Verification items for the finished model (mm, model axes). A direction names the side the tool comes from. Round coordinates to 2 decimals unless told otherwise and drop trailing zeros. Write each loop counter-clockwise with the first axis right and the second up, starting at its lowest first coordinate (ties: lowest second). Pieces come first, ordered by that corner, then holes. Notation, with made-up numbers: (-29, 62) -> (-11, 62) arc R17 cw to (-11, 90) -> close; hole circle Ø3 at (-16, 37). An arc over 180 degrees is marked (long way). Answer as a JSON object with one key per item and string values. Group by question number.
(1) Scan lines: L1, parallel to X at y = 1.05, z = 38.9; L2, parallel to X at y = 0.2, z = 32.5; L3, parallel to X at y = 2.85, z = 30 (3 decimals). Record each from-to range of solid material in increasing order. Write a range as from..to.
(2) Sectioned sample at A-A on x = -7.5. Record the cut outline in (y, z), and give its area (3 significant figures).
(3) Sectioned sample at C-C on z = 28.9. Record the cut outline in (x, y).
(4) Sectioned sample at B-B on x = -27.5. Record the cut outline in (y, z), and give its area (3 significant figures).
(5) Draft check along X on faces 1 (the face through (-1, 0, 12)), 2 (the face through (31, 1, 7.5)), 3 (the face through (50, 1, 1)). Enter one of: released by +X, released by -X, zero draft, split by the parting line, or undercut.
(6) Gauge pin test, flat end, axial feed: pin 1 Ø1 at (y, z) = (0.5, 13.5) entering from -X. Record the tip position at first contact, or that the pin passes through.
(7) Set-up check for faces 4 (the face through (12.5, 2, 25)), 5 (the face through (-50, 1, 1)): record each of +Z, -Z, +X, -X, +Y, -Y from which the full face is reachable in a straight line by a thin tool's end or side.
(8) Sectioned sample at D-D on x = 18.5. Record the cut outline in (y, z).
```python
from build123d import *

# Parameters (mm, degrees)
SKETCH_1_W          = 100
SKETCH_1_H          = 15
EXTRUDE_1_DEPTH     = 3
SKETCH_2_W          = 25
SKETCH_2_H          = 50
EXTRUDE_2_DEPTH     = 3
SKETCH_3_R          = 1.6
CUT_EXTRUDE_1_DEPTH = 3
EXTRUDE_3_DEPTH     = 3
CHAMFER_1_SIZE      = 10
FILLET_2_R          = 2


with BuildPart() as part:
    # 草图1 → 凸台-拉伸1 (new body)
    with BuildSketch(Plane(origin=(0, 0, 0), x_dir=(1, 0, 0), z_dir=(0, 1, 0))):
        Rectangle(SKETCH_1_W, SKETCH_1_H)
    extrude(amount=EXTRUDE_1_DEPTH)

    # 草图2 → 凸台-拉伸2 (add)
    with BuildSketch(Plane(origin=(0, 3, 0), x_dir=(1, 0, 0), z_dir=(0, 1, 0))):
        with Locations((0, -17.5)):
            Rectangle(SKETCH_2_W, SKETCH_2_H)
    extrude(amount=-EXTRUDE_2_DEPTH)

    # 草图3 → 切除-拉伸1 (cut)
    with BuildSketch(Plane(origin=(0, 3, 0), x_dir=(1, 0, 0), z_dir=(0, 1, 0))):
        with Locations(Location((-42.5, 3.75, 0), (0, 0, 270))):
            Circle(SKETCH_3_R)
        with Locations(Location((-42.5, -3.75, 0), (0, 0, 90))):
            Circle(SKETCH_3_R)
        with Locations(Location((-27.5, -3.75, 0), (0, 0, 270))):
            Circle(SKETCH_3_R)
        with Locations(Location((-27.5, 3.75, 0), (0, 0, 90))):
            Circle(SKETCH_3_R)
        with Locations(Location((27.5, -3.75, 0), (0, 0, 90))):
            Circle(SKETCH_3_R)
        with Locations(Location((42.5, -3.75, 0), (0, 0, 270))):
            Circle(SKETCH_3_R)
        with Locations(Location((42.5, 3.75, 0), (0, 0, 90))):
            Circle(SKETCH_3_R)
        with Locations(Location((27.5, 3.75, 0), (0, 0, 270))):
            Circle(SKETCH_3_R)
        with Locations(Location((-7.5, 5, 0), (0, 0, 270))):
            Circle(SKETCH_3_R)
        with Locations(Location((-7.5, -5, 0), (0, 0, 90))):
            Circle(SKETCH_3_R)
        with Locations(Location((7.5, -5, 0), (0, 0, 270))):
            Circle(SKETCH_3_R)
        with Locations(Location((7.5, 5, 0), (0, 0, 90))):
            Circle(SKETCH_3_R)
        with Locations(Location((-7.5, -28.9, 0), (0, 0, 270))):
            Circle(SKETCH_3_R)
        with Locations(Location((-7.5, -38.9, 0), (0, 0, 90))):
            Circle(SKETCH_3_R)
        with Locations(Location((7.5, -38.9, 0), (0, 0, 270))):
            Circle(SKETCH_3_R)
        with Locations(Location((7.5, -28.9, 0), (0, 0, 90))):
            Circle(SKETCH_3_R)
    extrude(amount=-CUT_EXTRUDE_1_DEPTH, mode=Mode.SUBTRACT)

    # 草图4 → 凸台-拉伸3 (add)
    with BuildSketch(Plane(origin=(0, 3, 0), x_dir=(1, 0, 0), z_dir=(0, 1, 0))):
        Polygon((-50, -7.5), (-12.5, -42.5), (-12.5, -37.5), (-45, -7.5), align=None)
        Polygon((12.5, -37.5), (45, -7.5), (50, -7.5), (12.5, -42.5), align=None)
    extrude(amount=-EXTRUDE_3_DEPTH)

    # 倒角1
    chamfer_1_edges = [part.edges().sort_by_distance(p)[0] for p in [
        (-12.5, 1.5, 7.5),
        (12.5, 1.5, 7.5),
    ]]
    chamfer(chamfer_1_edges, length=CHAMFER_1_SIZE)

    # 圆角2
    fillet_2_edges = [part.edges().sort_by_distance(p)[0] for p in [
        (-45, 1.5, 7.5),
        (-12.5, 1.5, 37.5),
        (12.5, 1.5, 37.5),
        (45, 1.5, 7.5),
        (-50, 1.5, -7.5),
        (50, 1.5, -7.5),
    ]]
    fillet(fillet_2_edges, radius=FILLET_2_R)


solid = part.part
```
Computed values:
{
 "1": {"L1": "-16.36..-9.1, -5.9..5.9, 9.1..16.36", "L2": "-23.21..-17.92, -12.5..12.5, 17.92..23.21", "L3": "-25.893..-20.625, -12.5..-8.662, -6.338..6.338, 8.662..12.5, 20.625..25.893"},
 "2": {"outline": "(0, -7.5) -> (3, -7.5) -> (3, -6.6) -> (0, -6.6) -> close; (0, -3.4) -> (3, -3.4) -> (3, 3.4) -> (0, 3.4) -> close; (0, 6.6) -> (3, 6.6) -> (3, 27.3) -> (0, 27.3) -> close; (0, 30.5) -> (3, 30.5) -> (3, 37.3) -> (0, 37.3) -> close; (0, 40.5) -> (3, 40.5) -> (3, 42.5) -> (0, 42.5) -> close", "area": "112 mm2"},
 "3": {"outline": "(-27.07, 0) -> (-21.82, 0) -> (-21.82, 3) -> (-27.07, 3) -> close; (-12.5, 0) -> (-9.1, 0) -> (-9.1, 3) -> (-12.5, 3) -> close; (-5.9, 0) -> (5.9, 0) -> (5.9, 3) -> (-5.9, 3) -> close; (9.1, 0) -> (12.5, 0) -> (12.5, 3) -> (9.1, 3) -> close; (21.82, 0) -> (27.07, 0) -> (27.07, 3) -> (21.82, 3) -> close"},
 "4": {"outline": "(0, -7.5) -> (3, -7.5) -> (3, -5.35) -> (0, -5.35) -> close; (0, -2.15) -> (3, -2.15) -> (3, 2.15) -> (0, 2.15) -> close; (0, 5.35) -> (3, 5.35) -> (3, 7.5) -> (0, 7.5) -> close; (0, 23.65) -> (3, 23.65) -> (3, 28.5) -> (0, 28.5) -> close", "area": "40.3 mm2"},
 "5": {"face 1": "zero draft", "face 2": "undercut", "face 3": "released by +X"},
 "6": {"pin 1": "x = -44.11"},
 "7": {"face 4": "+Y, -Y", "face 5": "+Z, -Z, -X, +Y, -Y"},
 "8": {"outline": "(0, -7.5) -> (3, -7.5) -> (3, 11.5) -> (0, 11.5) -> close; (0, 31.96) -> (3, 31.96) -> (3, 36.9) -> (0, 36.9) -> close"}
}
